Read the model definition and answer for the solid it produces. Units are mm, in the model's axes. Coordinates: 2 decimals unless noted, no trailing zeros. Loops run counter-clockwise (first coordinate to the right, second up) from the corner with the lowest first, then second, coordinate; pieces in that order, holes last. Notation, with made-up numbers: M -39,26.25 L -8,26.25 A27 ccw -8,59.25 Z; hole C 46.5,-1.5 d3. An arc over 180 degrees is marked long. Use one line per item in the form item = value. Start each with the question number.
1. The part is cut by section B-B (y = 0.8). Give the number of separate pieces and of enclosed holes in the cut face, plus the area to 3 significant figures.
2. Find the intervals of material crossed by probe 1 along Z at (x, y) = (-28, 0.35); probe 2 along Z at (x, y) = (-45, 1.15); probe 3 along Z at (x, y) = (0.5, 1.35), in increasing order. Write a range as [from, to].
3. Flat-ended cylindrical pins translate along their axes: pin 1 (0.5 mm diameter, centred on x = -4.5, y = 1, fed in from +Z); pin 2 (0.5 mm diameter, centred on x = -1, y = 1.5, fed in from +Z); pin 3 (2.5 mm diameter, centred on x = 46.35, z = -32.14, fed in from +Y) (3 decimals). Find the tip coordinate at first contact, or state that the pin passes through.
4. The part is cut by section A-A (x = 41.25). Give the vertices of the cut face in (y, z).
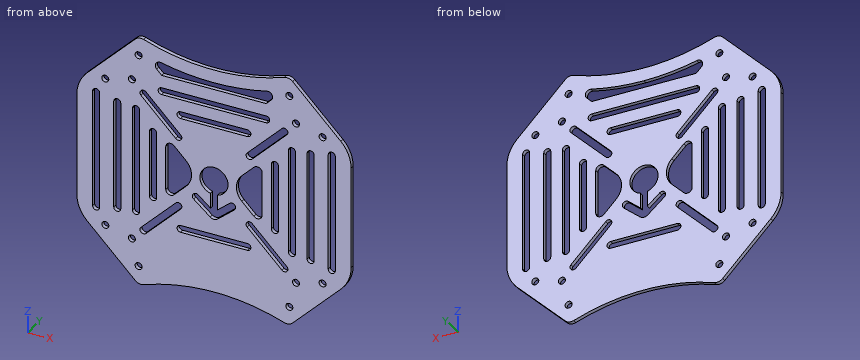
from build123d import *

# Parameters (mm, degrees)
SKETCH_1_R      = 1.5
EXTRUDE_1_DEPTH = 1.7
FILLET_1_R      = 3.5
FILLET_2_R      = 15


with BuildPart() as part:
    # 草圖1 → 填料-伸長1 (new body)
    with BuildSketch(Plane(origin=(0, 0, 0), x_dir=(1, 0, 0), z_dir=(0, 1, 0))):
        with BuildLine():
            Line((-31.988251141, -54.632329554), (-58.5, -28.120580695))
            Line((-58.5, -28.120580695), (-58.5, 28.120580695))
            Line((-58.5, 28.120580695), (-31.988251141, 54.632329554))
            ThreePointArc((-31.988251141, 54.632329554), (0, 48.75576142), (31.988251141, 54.632329554))
            Line((31.988251141, 54.632329554), (58.5, 28.120580695))
            Line((58.5, 28.120580695), (58.5, -28.120580695))
            Line((58.5, -28.120580695), (31.988251141, -54.632329554))
            ThreePointArc((31.988251141, -54.632329554), (0, -48.75576142), (-31.988251141, -54.632329554))
        make_face()
        with Locations((-35.001785669, 35.001785669)):
            Circle(SKETCH_1_R, mode=Mode.SUBTRACT)
        with Locations((35.001785669, -35.001785669)):
            Circle(SKETCH_1_R, mode=Mode.SUBTRACT)
        with Locations((-35.001785669, -35.001785669)):
            Circle(SKETCH_1_R, mode=Mode.SUBTRACT)
        with Locations((35.001785669, 35.001785669)):
            Circle(SKETCH_1_R, mode=Mode.SUBTRACT)
        with Locations((-32.138003205, -46.350849507)):
            Circle(SKETCH_1_R, mode=Mode.SUBTRACT)
        with Locations((-46.350849507, -32.138003205)):
            Circle(SKETCH_1_R, mode=Mode.SUBTRACT)
        with Locations((-32.138003205, 46.350849507)):
            Circle(SKETCH_1_R, mode=Mode.SUBTRACT)
        with Locations((-46.350849507, 32.138003205)):
            Circle(SKETCH_1_R, mode=Mode.SUBTRACT)
        with Locations((46.350849507, 32.138003205)):
            Circle(SKETCH_1_R, mode=Mode.SUBTRACT)
        with Locations((32.138003205, 46.350849507)):
            Circle(SKETCH_1_R, mode=Mode.SUBTRACT)
        with Locations((32.138003205, -46.350849507)):
            Circle(SKETCH_1_R, mode=Mode.SUBTRACT)
        with Locations((46.350849507, -32.138003205)):
            Circle(SKETCH_1_R, mode=Mode.SUBTRACT)
        with BuildLine():
            Line((-14.25, 26.5), (14.25, 26.5))
            ThreePointArc((14.25, 26.5), (15.75, 25), (14.25, 23.5))
            Line((14.25, 23.5), (-14.25, 23.5))
            ThreePointArc((-14.25, 23.5), (-15.75, 25), (-14.25, 26.5))
        make_face(mode=Mode.SUBTRACT)
        with BuildLine():
            Line((-14.25, -26.5), (14.25, -26.5))
            ThreePointArc((14.25, -26.5), (15.75, -25), (14.25, -23.5))
            Line((14.25, -23.5), (-14.25, -23.5))
            ThreePointArc((-14.25, -23.5), (-15.75, -25), (-14.25, -26.5))
        make_face(mode=Mode.SUBTRACT)
        with BuildLine():
            Line((-28.991378029, 31.112698372), (-14.142135624, 16.263455967))
            ThreePointArc((-14.142135624, 16.263455967), (-14.142135624, 14.142135624), (-16.263455967, 14.142135624))
            Line((-16.263455967, 14.142135624), (-31.112698372, 28.991378029))
            ThreePointArc((-31.112698372, 28.991378029), (-31.112698372, 31.112698372), (-28.991378029, 31.112698372))
        make_face(mode=Mode.SUBTRACT)
        with BuildLine():
            Line((28.991378029, 31.112698372), (14.142135624, 16.263455967))
            ThreePointArc((14.142135624, 16.263455967), (14.142135624, 14.142135624), (16.263455967, 14.142135624))
            Line((16.263455967, 14.142135624), (31.112698372, 28.991378029))
            ThreePointArc((31.112698372, 28.991378029), (31.112698372, 31.112698372), (28.991378029, 31.112698372))
        make_face(mode=Mode.SUBTRACT)
        with BuildLine():
            Line((28.991378029, -31.112698372), (14.142135624, -16.263455967))
            ThreePointArc((14.142135624, -16.263455967), (14.142135624, -14.142135624), (16.263455967, -14.142135624))
            Line((16.263455967, -14.142135624), (31.112698372, -28.991378029))
            ThreePointArc((31.112698372, -28.991378029), (31.112698372, -31.112698372), (28.991378029, -31.112698372))
        make_face(mode=Mode.SUBTRACT)
        with BuildLine():
            Line((-28.991378029, -31.112698372), (-14.142135624, -16.263455967))
            ThreePointArc((-14.142135624, -16.263455967), (-14.142135624, -14.142135624), (-16.263455967, -14.142135624))
            Line((-16.263455967, -14.142135624), (-31.112698372, -28.991378029))
            ThreePointArc((-31.112698372, -28.991378029), (-31.112698372, -31.112698372), (-28.991378029, -31.112698372))
        make_face(mode=Mode.SUBTRACT)
        with BuildLine():
            Line((-31.75, 22.4), (-31.75, -22.4))
            ThreePointArc((-31.75, -22.4), (-33.25, -23.9), (-34.75, -22.4))
            Line((-34.75, -22.4), (-34.75, 22.4))
            ThreePointArc((-34.75, 22.4), (-33.25, 23.9), (-31.75, 22.4))
        make_face(mode=Mode.SUBTRACT)
        with BuildLine():
            Line((-39.75, 23.25), (-39.75, -23.25))
            ThreePointArc((-39.75, -23.25), (-41.25, -24.75), (-42.75, -23.25))
            Line((-42.75, -23.25), (-42.75, 23.25))
            ThreePointArc((-42.75, 23.25), (-41.25, 24.75), (-39.75, 23.25))
        make_face(mode=Mode.SUBTRACT)
        with BuildLine():
            Line((-48.75, 25.2), (-48.75, -25.2))
            ThreePointArc((-48.75, -25.2), (-50.25, -26.7), (-51.75, -25.2))
            Line((-51.75, -25.2), (-51.75, 25.2))
            ThreePointArc((-51.75, 25.2), (-50.25, 26.7), (-48.75, 25.2))
        make_face(mode=Mode.SUBTRACT)
        with BuildLine():
            Line((48.75, 25.2), (48.75, -25.2))
            ThreePointArc((48.75, -25.2), (50.25, -26.7), (51.75, -25.2))
            Line((51.75, -25.2), (51.75, 25.2))
            ThreePointArc((51.75, 25.2), (50.25, 26.7), (48.75, 25.2))
        make_face(mode=Mode.SUBTRACT)
        with BuildLine():
            Line((39.75, 23.25), (39.75, -23.25))
            ThreePointArc((39.75, -23.25), (41.25, -24.75), (42.75, -23.25))
            Line((42.75, -23.25), (42.75, 23.25))
            ThreePointArc((42.75, 23.25), (41.25, 24.75), (39.75, 23.25))
        make_face(mode=Mode.SUBTRACT)
        with BuildLine():
            Line((31.75, 22.4), (31.75, -22.4))
            ThreePointArc((31.75, -22.4), (33.25, -23.9), (34.75, -22.4))
            Line((34.75, -22.4), (34.75, 22.4))
            ThreePointArc((34.75, 22.4), (33.25, 23.9), (31.75, 22.4))
        make_face(mode=Mode.SUBTRACT)
        with BuildLine():
            Line((-24.5, 14.3), (-24.5, -14.3))
            ThreePointArc((-24.5, -14.3), (-26, -15.8), (-27.5, -14.3))
            Line((-27.5, -14.3), (-27.5, 14.3))
            ThreePointArc((-27.5, 14.3), (-26, 15.8), (-24.5, 14.3))
        make_face(mode=Mode.SUBTRACT)
        with BuildLine():
            Line((-1.5, 5.809475019), (-1.5, 12.309475019))
            Line((-1.5, 12.309475019), (-6.701273653, 7.945088216))
            ThreePointArc((-6.701273653, 7.945088216), (-8.884963334, 8.136136308), (-8.693915243, 10.319825989))
            Line((-8.693915243, 10.319825989), (-1.606969024, 16.266479947))
            ThreePointArc((-1.606969024, 16.266479947), (0, 16.85136884), (1.606969024, 16.266479947))
            Line((1.606969024, 16.266479947), (8.693915243, 10.319825989))
            ThreePointArc((8.693915243, 10.319825989), (8.884963334, 8.136136308), (6.701273653, 7.945088216))
            Line((6.701273653, 7.945088216), (1.5, 12.309475019))
            Line((1.5, 12.309475019), (1.5, 5.809475019))
            ThreePointArc((1.5, 5.809475019), (0, -6), (-1.5, 5.809475019))
        make_face(mode=Mode.SUBTRACT)
        with BuildLine():
            Line((24.5, 14.3), (24.5, -14.3))
            ThreePointArc((24.5, -14.3), (26, -15.8), (27.5, -14.3))
            Line((27.5, -14.3), (27.5, 14.3))
            ThreePointArc((27.5, 14.3), (26, 15.8), (24.5, 14.3))
        make_face(mode=Mode.SUBTRACT)
        with BuildLine():
            Line((-22.3, -31.8), (22.3, -31.8))
            ThreePointArc((22.3, -31.8), (23.8, -33.3), (22.3, -34.8))
            Line((22.3, -34.8), (-22.3, -34.8))
            ThreePointArc((-22.3, -34.8), (-23.8, -33.3), (-22.3, -31.8))
        make_face(mode=Mode.SUBTRACT)
        with BuildLine():
            Line((20.566347785, -9.367820826), (20.566347785, 9.367820826))
            ThreePointArc((20.566347785, 9.367820826), (19.303516728, 11.257781063), (17.074156624, 10.814333767))
            Line((17.074156624, 10.814333767), (11.904413984, 5.644591127))
            ThreePointArc((11.904413984, 5.644591127), (9.566347785, 0), (11.904413984, -5.644591127))
            Line((11.904413984, -5.644591127), (17.074156624, -10.814333767))
            ThreePointArc((17.074156624, -10.814333767), (19.303516728, -11.257781063), (20.566347785, -9.367820826))
        make_face(mode=Mode.SUBTRACT)
        with BuildLine():
            Line((-17.074156624, -10.814333767), (-11.904413984, -5.644591127))
            ThreePointArc((-11.904413984, -5.644591127), (-9.566347785, 0), (-11.904413984, 5.644591127))
            Line((-11.904413984, 5.644591127), (-17.074156624, 10.814333767))
            ThreePointArc((-17.074156624, 10.814333767), (-19.303516728, 11.257781063), (-20.566347785, 9.367820826))
            Line((-20.566347785, 9.367820826), (-20.566347785, -9.367820826))
            ThreePointArc((-20.566347785, -9.367820826), (-19.303516728, -11.257781063), (-17.074156624, -10.814333767))
        make_face(mode=Mode.SUBTRACT)
        with BuildLine():
            Line((-22.261855959, -40.237571716), (22.261855959, -40.237571716))
            Line((22.261855959, -40.237571716), (24.43166791, -42.407383666))
            ThreePointArc((24.43166791, -42.407383666), (24.766340216, -44.791854009), (22.566131713, -45.770008859))
            ThreePointArc((22.566131713, -45.770008859), (11.356536667, -43.837537687), (0, -43.190590357))
            ThreePointArc((0, -43.190590357), (-11.356536667, -43.837537687), (-22.566131713, -45.770008859))
            ThreePointArc((-22.566131713, -45.770008859), (-24.766340216, -44.791854009), (-24.43166791, -42.407383666))
            Line((-24.43166791, -42.407383666), (-22.261855959, -40.237571716))
        make_face(mode=Mode.SUBTRACT)
    extrude(amount=EXTRUDE_1_DEPTH)

    # 圓角1
    fillet_1_edges = [part.edges().sort_by_distance(p)[0] for p in [
        (31.988251141, 0.85, 54.632329554),
        (-31.988251141, 0.85, 54.632329554),
        (-31.988251141, 0.85, -54.632329554),
        (31.988251141, 0.85, -54.632329554),
    ]]
    fillet(fillet_1_edges, radius=FILLET_1_R)

    # 圓角2
    fillet_2_edges = [part.edges().sort_by_distance(p)[0] for p in [
        (58.5, 0.85, -28.120580695),
        (58.5, 0.85, 28.120580695),
        (-58.5, 0.85, 28.120580695),
        (-58.5, 0.85, -28.120580695),
    ]]
    fillet(fillet_2_edges, radius=FILLET_2_R)


solid = part.part
Computed values:
q1.separate_pieces = 1
q1.enclosed_holes = 31
q1.area = 8,330 mm²
q2.probe_1 = [-53.22, -30.12], [-25.88, 25.88], [30.12, 53.22]
q2.probe_2 = [-41.62, -32.79], [-31.49, 31.49], [32.79, 41.62]
q2.probe_3 = [-48.76, -26.5], [-23.5, -16.8], [5.98, 23.5], [26.5, 31.8], [34.8, 40.24], [43.19, 48.76]
q3.pin_1 = 48.88
q3.pin_2 = 48.76
q3.pin_3 = through
q4.outline = M 0,-45.37 L 1.7,-45.37 L 1.7,-24.75 L 0,-24.75 Z; M 0,24.75 L 1.7,24.75 L 1.7,45.37 L 0,45.37 Z
